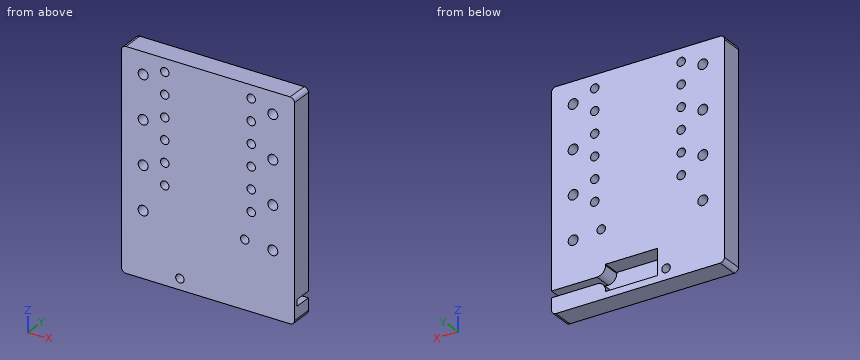
```python
from build123d import *

# Parameters (mm, degrees)
SKETCH1_W           = 40
SKETCH1_H           = 50
BOSS_EXTRUDE1_DEPTH = 5
SKETCH9_R           = 1.15
CUT_EXTRUDE8_DEPTH  = 33.403703492
LPATTERN2_COUNT     = 3
LPATTERN2_PITCH     = 10
LPATTERN2_COL_COUNT = 2
LPATTERN2_COL_PITCH = 10
SKETCH4_R           = 0.975
CUT_EXTRUDE3_DEPTH  = 33.403703492
SKETCH5_R           = 0.975
CUT_EXTRUDE4_DEPTH  = 33.403703492
LPATTERN1_COUNT     = 6
LPATTERN1_PITCH     = 5
FILLET1_R           = 1
CUT_EXTRUDE7_DEPTH  = 4
FILLET2_R           = 2


with BuildPart() as part:
    # Sketch1 → Boss-Extrude1 (new body)
    with BuildSketch(Plane(origin=(0, 0, 0), x_dir=(1, 0, 0), z_dir=(0, 1, 0))):
        Rectangle(SKETCH1_W, SKETCH1_H)
    extrude(amount=BOSS_EXTRUDE1_DEPTH)

    # Sketch9 → Cut-Extrude8 (cut, through all)
    with BuildSketch(Plane(origin=(0, 5, 0), x_dir=(1, 0, 0), z_dir=(0, 1, 0))):
        with Locations(Location((-15, 0, 0), (0, 0, 270))):
            Circle(SKETCH9_R)
        with Locations(Location((15, 0, 0), (0, 0, 90))):
            Circle(SKETCH9_R)
    cut_extrude8 = extrude(amount=-CUT_EXTRUDE8_DEPTH, mode=Mode.SUBTRACT)

    # LPattern2: Cut-Extrude8 ×3
    with Locations(*[(0, 0, i * LPATTERN2_PITCH) for i in range(1, LPATTERN2_COUNT)]):
        add(cut_extrude8, mode=Mode.SUBTRACT)

    # LPattern2 col: Cut-Extrude8 ×2
    with Locations(*[(0, 0, -i * LPATTERN2_COL_PITCH) for i in range(1, LPATTERN2_COL_COUNT)]):
        add(cut_extrude8, mode=Mode.SUBTRACT)

    # Sketch4 → Cut-Extrude3 (cut, through all)
    with BuildSketch(Plane(origin=(0, 5, 0), x_dir=(1, 0, 0), z_dir=(0, 1, 0))):
        with Locations(Location((-6.5, 22.5, 0), (0, 0, 270))):
            Circle(SKETCH4_R)
        with Locations(Location((8.5, 9.5, 0), (0, 0, 270))):
            Circle(SKETCH4_R)
    extrude(amount=-CUT_EXTRUDE3_DEPTH, mode=Mode.SUBTRACT)

    # Sketch5 → Cut-Extrude4 (cut, through all)
    with BuildSketch(Plane(origin=(0, 5, 0), x_dir=(1, 0, 0), z_dir=(0, 1, 0))):
        with Locations(Location((-10, -22, 0), (0, 0, 270))):
            Circle(SKETCH5_R)
        with Locations(Location((10, -22, 0), (0, 0, 90))):
            Circle(SKETCH5_R)
    cut_extrude4 = extrude(amount=-CUT_EXTRUDE4_DEPTH, mode=Mode.SUBTRACT)

    # LPattern1: Cut-Extrude4 ×6
    with Locations(*[(0, 0, -i * LPATTERN1_PITCH) for i in range(1, LPATTERN1_COUNT)]):
        add(cut_extrude4, mode=Mode.SUBTRACT)

    # Fillet1
    fillet1_edges = [part.edges().sort_by_distance(p)[0] for p in [
        (20, 2.5, 25),
        (-20, 2.5, 25),
        (-20, 2.5, -25),
        (20, 2.5, -25),
    ]]
    fillet(fillet1_edges, radius=FILLET1_R)

    # Sketch8 → Cut-Extrude7 (cut)
    with BuildSketch(Plane(origin=(0, 5, 0), x_dir=(1, 0, 0), z_dir=(0, 1, 0))):
        Polygon((7.5, 23.5), (7.5, 21.25), (20, 21.25), (20, 19.75), (7.5, 19.75), (7.5, 17.5), (-4.5, 17.5), (-4.5, 23.5), align=None)
    extrude(amount=-CUT_EXTRUDE7_DEPTH, mode=Mode.SUBTRACT)

    # Fillet2
    fillet2_edges = [part.edges().sort_by_distance(p)[0] for p in [
        (7.5, 3, -19.75),
        (7.5, 3, -21.25),
    ]]
    fillet(fillet2_edges, radius=FILLET2_R)


solid = part.part
```
Geometry check sheet. Reference: the model listing, model coordinates, mm. Coordinates: 2 decimals unless noted, no trailing zeros. Order: outer loops, then holes, each group sorted by start corner. A loop starts at its lowest first (then second) coordinate and runs counter-clockwise, first axis right, second up. Notation, with made-up numbers: (11.25, 59.25) - (28.25, 59.25) arc R7 ccw to (28.25, 65.25) - close; hole circle Ø3 at (-11.75, -17.75). An arc over 180 degrees is marked (long way). Answer in a Markdown table with one row per item. Add a question column.
1. Section check D-D (x = 1.5). Enter the section's corners in (y, z).
2. Section check C-C (x = -10). Enter the section's corners in (y, z) (3 decimals).
3. Material ranges on L1, parallel to X at y = 1.35, z = 0; L2, parallel to X at y = 2.7, z = 2 (3 decimals); L3, parallel to Z at x = 15.5, y = 4.6, recorded low to high. Write a range as [from, to].
4. Section check A-A (z = 2). Enter the section's corners in (x, y) (3 decimals).
5. Section check B-B (x = -15). Enter the section's corners in (y, z).
Data:
| question | item | result |
|---|---|---|
| 1 | outline | (0, -25) - (5, -25) - (5, -23.5) - (1, -23.5) - (1, -17.5) - (5, -17.5) - (5, 25) - (0, 25) - close |
| 2 | outline | (0, -25) - (5, -25) - (5, -3.975) - (0, -3.975) - close; (0, -2.025) - (5, -2.025) - (5, 1.025) - (0, 1.025) - close; (0, 2.975) - (5, 2.975) - (5, 6.025) - (0, 6.025) - close; (0, 7.975) - (5, 7.975) - (5, 11.025) - (0, 11.025) - close; (0, 12.975) - (5, 12.975) - (5, 16.025) - (0, 16.025) - close; (0, 17.975) - (5, 17.975) - (5, 21.025) - (0, 21.025) - close; (0, 22.975) - (5, 22.975) - (5, 25) - (0, 25) - close |
| 3 | L1 | x = [-20, -16.15], [-13.85, 13.85], [16.15, 20] |
| 3 | L2 | x = [-20, -10.975], [-9.025, 9.025], [10.975, 20] |
| 3 | L3 | z = [-25, -21.25], [-19.75, -11.04], [-8.96, -1.04], [1.04, 8.96], [11.04, 18.96], [21.04, 25] |
| 4 | outline | (-20, 0) - (-10.975, 0) - (-10.975, 5) - (-20, 5) - close; (-9.025, 0) - (9.025, 0) - (9.025, 5) - (-9.025, 5) - close; (10.975, 0) - (20, 0) - (20, 5) - (10.975, 5) - close |
| 5 | outline | (0, -25) - (5, -25) - (5, -11.15) - (0, -11.15) - close; (0, -8.85) - (5, -8.85) - (5, -1.15) - (0, -1.15) - close; (0, 1.15) - (5, 1.15) - (5, 8.85) - (0, 8.85) - close; (0, 11.15) - (5, 11.15) - (5, 18.85) - (0, 18.85) - close; (0, 21.15) - (5, 21.15) - (5, 25) - (0, 25) - close |
